For this review, take the finished solid that the model builds, in its own axes (mm). Give positions to 0.01 mm unless a question says otherwise; leave off trailing zeros. Order: outer loops, then holes, each group sorted by start corner. A loop starts at its lowest first (then second) coordinate and runs counter-clockwise, first axis right, second up. Notation, with made-up numbers: (7, 88.5) - (25, 88.5) arc R27 cw to (25, 122.5) - close; hole circle Ø11 at (3, 33.25). An arc over 180 degrees is marked (long way). Put each result on its own line as item: value. Start each with the question number.
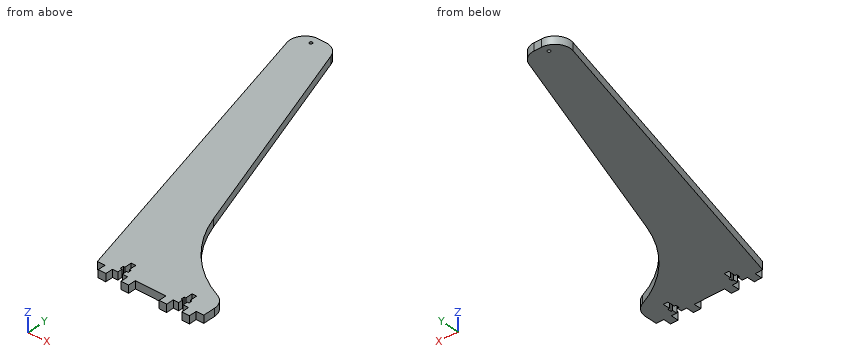
```python
from build123d import *

# Parameters (mm, degrees)
BOSS_EXTRU_1_OUTLINE_R = 1
BOSS_EXTRU_1_DEPTH     = 5
CONG_1_R               = 10


# Read off the part's stored shape, not the designer's step: Boss.-Extru.1
with BuildPart() as part:
    # Boss.-Extru.1 outline → Boss.-Extru.1 (new body)
    with BuildSketch(Plane.XY):
        with BuildLine():
            Line((-67.5, 216), (-92.5, 216))
            Line((-92.5, 216), (-35, 0))
            Line((-35, 0), (-30, 0))
            Line((-30, 0), (-30, -5))
            Line((-30, -5), (-25, -5))
            Line((-25, -5), (-25, 0))
            Line((-25, 0), (-21.5, 0))
            Line((-21.5, 0), (-21.5, 3))
            Line((-21.5, 3), (-22.6, 3))
            Line((-22.6, 3), (-22.6, 5.3))
            Line((-22.6, 5.3), (-21.5, 5.3))
            Line((-21.5, 5.3), (-21.5, 10))
            Line((-21.5, 10), (-18.5, 10))
            Line((-18.5, 10), (-18.5, 5.3))
            Line((-18.5, 5.3), (-17.4, 5.3))
            Line((-17.4, 5.3), (-17.4, 3))
            Line((-17.4, 3), (-18.5, 3))
            Line((-18.5, 3), (-18.5, 0))
            Line((-18.5, 0), (-15, 0))
            Line((-15, 0), (-15, -5))
            Line((-15, -5), (-10, -5))
            Line((-10, -5), (-10, 0))
            Line((-10, 0), (10, 0))
            Line((10, 0), (10, -5))
            Line((10, -5), (15, -5))
            Line((15, -5), (15, 0))
            Line((15, 0), (18.5, 0))
            Line((18.5, 0), (18.5, 3))
            Line((18.5, 3), (17.4, 3))
            Line((17.4, 3), (17.4, 5.3))
            Line((17.4, 5.3), (18.5, 5.3))
            Line((18.5, 5.3), (18.5, 10))
            Line((18.5, 10), (21.5, 10))
            Line((21.5, 10), (21.5, 5.3))
            Line((21.5, 5.3), (22.6, 5.3))
            Line((22.6, 5.3), (22.6, 3))
            Line((22.6, 3), (21.5, 3))
            Line((21.5, 3), (21.5, 0))
            Line((21.5, 0), (25, 0))
            Line((25, 0), (25, -5))
            Line((25, -5), (30, -5))
            Line((30, -5), (30, 0))
            Line((30, 0), (35, 0))
            Line((35, 0), (35, 15))
            ThreePointArc((35, 15), (3.448702598, 34.108667771), (-16.175379452, 65.341998613))
            Line((-16.175379452, 65.341998613), (-67.5, 216))
        make_face()
        with Locations((-80, 211)):
            Circle(BOSS_EXTRU_1_OUTLINE_R, mode=Mode.SUBTRACT)
    extrude(amount=BOSS_EXTRU_1_DEPTH)

    # Congé1
    cong_1_edges = [part.edges().sort_by_distance(p)[0] for p in [
        (-67.5, 216, 2.5),
        (35, 15, 2.5),
        (-92.5, 216, 2.5),
    ]]
    fillet(cong_1_edges, radius=CONG_1_R)


solid = part.part
```
1. Add section B-B, the plane y = 151. Give the boundary of the cut face in (x, z).
2. Clearance check with flat-ended pins moving along their axes: pin 1 (1.5 mm diameter, centred on y = -3.5, z = 2, fed in from +X); pin 2 (1 mm diameter, centred on y = 42, z = 1, fed in from -X); pin 3 (2.5 mm diameter, centred on x = -32, z = 2, fed in from -Y). State where each tip first meets the part, or that it passes through.
3. Add section A-A, the plane x = -27.5. Give the boundary of the cut face in (y, z), then the cut area to 3 significant figures.
4. Wall thickness on line 1 (X direction, y = 6.5, z = 1); line 2 (X direction, y = 211, z = 2.3); line 3 (X direction, y = 65, z = 2.75): over which ranges is each line inside the solid? List them lowest first. Write a range as from..to.
Found:
1. outline: (-75.2, 0) - (-45.36, 0) - (-45.36, 5) - (-75.2, 5) - close
2. pin 1: stops at x = 30
2. pin 2: stops at x = -46.31
2. pin 3: stops at y = 0
3. outline: (-5, 0) - (98.58, 0) - (98.58, 5) - (-5, 5) - close
3. area: 518 mm^2
4. line 1: x = -36.73..-21.5, -18.5..18.5, 21.5..35
4. line 2: x = -88.15..-81, -79..-66
4. line 3: x = -52.3..-16.06
